```python
from build123d import *

# Parameters (mm, degrees)
EXTRUDE1_DEPTH     = 1.2
SKETCH3_R          = 6.35
EXTRUDE2_DEPTH     = 1.5
EXTRUDE3_DEPTH     = 0.75
SKETCH5_R          = 0.75
EXTRUDE4_DEPTH     = 0.3
SKETCH7_W          = 1.2
SKETCH7_H          = 1.2
SCALE1_SCALE       = 0.5
CUT_EXTRUDE1_DEPTH = 0.001


with BuildPart() as part:
    # Sketch1 → Revolve1 (revolve)
    with BuildSketch(Plane.XY):
        with BuildLine():
            Line((0, 0), (-6.25, 0))
            Line((-6.25, 0), (-6.25, 2.751471863))
            ThreePointArc((-6.25, 2.751471863), (-6.20432772, 2.981081922), (-6.074264069, 3.175735931))
            Line((-6.074264069, 3.175735931), (-5.674264069, 3.575735931))
            ThreePointArc((-5.674264069, 3.575735931), (-5.498528137, 4), (-5.674264069, 4.424264069))
            Line((-5.674264069, 4.424264069), (-6.074264069, 4.824264069))
            ThreePointArc((-6.074264069, 4.824264069), (-6.20432772, 5.018918078), (-6.25, 5.248528137))
            Line((-6.25, 5.248528137), (-6.25, 10.6))
            ThreePointArc((-6.25, 10.6), (-6.132842712, 10.882842712), (-5.85, 11))
            Line((-5.85, 11), (0, 11))
            Line((0, 11), (0, 0))
        make_face()
    revolve(axis=Axis((0, 11, 0), (0, -1, 0)))

    # Sketch2 → Extrude1 (add)
    with BuildSketch(Plane.XZ):
        with BuildLine():
            Line((-6.5, 5.5), (-5.5, 6.5))
            Line((-5.5, 6.5), (-1, 6.5))
            Line((-1, 6.5), (-1, 1.6))
            Line((-1, 1.6), (1, 1.6))
            Line((1, 1.6), (1, 6.5))
            Line((1, 6.5), (5.5, 6.5))
            Line((5.5, 6.5), (6.5, 5.5))
            Line((6.5, 5.5), (6.5, -5.5))
            ThreePointArc((6.5, -5.5), (6.207106781, -6.207106781), (5.5, -6.5))
            Line((5.5, -6.5), (1, -6.5))
            Line((1, -6.5), (1, -1.6))
            Line((1, -1.6), (-1, -1.6))
            Line((-1, -1.6), (-1, -6.5))
            Line((-1, -6.5), (-5.5, -6.5))
            ThreePointArc((-5.5, -6.5), (-6.207106781, -6.207106781), (-6.5, -5.5))
            Line((-6.5, -5.5), (-6.5, 5.5))
        make_face()
    extrude(amount=EXTRUDE1_DEPTH)

    # Sketch3 → Extrude2 (add)
    with BuildSketch(Plane(origin=(0, 0, 0), x_dir=(1, 0, 0), z_dir=(0, 1, 0))):
        with BuildLine():
            Line((5.5, -6.5), (-5.5, -6.5))
            Line((-5.5, -6.5), (-6.5, -5.5))
            Line((-6.5, -5.5), (-6.5, 5.5))
            ThreePointArc((-6.5, 5.5), (-6.207106781, 6.207106781), (-5.5, 6.5))
            Line((-5.5, 6.5), (5.5, 6.5))
            ThreePointArc((5.5, 6.5), (6.207106781, 6.207106781), (6.5, 5.5))
            Line((6.5, 5.5), (6.5, -5.5))
            Line((6.5, -5.5), (5.5, -6.5))
        make_face()
        Circle(SKETCH3_R, mode=Mode.SUBTRACT)
    extrude(amount=EXTRUDE2_DEPTH)

    # Sketch4 → Extrude3 (cut)
    with BuildSketch(Plane(origin=(0, 1.5, 0), x_dir=(1, 0, 0), z_dir=(0, 1, 0))):
        with BuildLine():
            Line((-6.5, 0), (-6.35, 0))
            ThreePointArc((-6.35, 0), (0, -6.35), (6.35, 0))
            Line((6.35, 0), (6.5, 0))
            Line((6.5, 0), (6.5, -5.5))
            Line((6.5, -5.5), (5.5, -6.5))
            Line((5.5, -6.5), (-5.5, -6.5))
            Line((-5.5, -6.5), (-6.5, -5.5))
            Line((-6.5, -5.5), (-6.5, 0))
        make_face()
    extrude(amount=-EXTRUDE3_DEPTH, mode=Mode.SUBTRACT)

    # Sketch5 → Extrude4 (add)
    with BuildSketch(Plane.XZ.offset(1.2)):
        with Locations((-4, 4)):
            Circle(SKETCH5_R)
        with Locations((4, 4)):
            Circle(SKETCH5_R)
        with Locations((-4, -4)):
            Circle(SKETCH5_R)
        with Locations((4, -4)):
            Circle(SKETCH5_R)
    extrude(amount=EXTRUDE4_DEPTH)

    # Sweep1: sweep along a path in Sketch6
    with BuildLine(Plane(origin=(0, 0, 0), x_dir=(0, 0, -1), z_dir=(1, 0, 0))) as sweep1_path:
        Line((2.7, 0), (2.7, -0.05))
        ThreePointArc((2.7, -0.05), (3.051471863, -0.898528137), (3.9, -1.25))
        Line((3.9, -1.25), (6.85, -1.25))
    # Sketch7 → Sweep1 (sweep)
    with BuildSketch(Plane.XZ):
        with Locations((0, -2.7)):
            Rectangle(SKETCH7_W, SKETCH7_H)
    sweep1 = sweep(path=sweep1_path.line)

    # Mirror1: Sweep1 across plane
    add(sweep1.mirror(Plane.XY))


with BuildPart() as part_1:
    # Scale1: scaled about (0, 4.617982794, -0.053235297)
    add(part.part.scale(SCALE1_SCALE).moved(Location((0, 2.308991397, -0.026617649))))

    # Sketch8 → Cut-Extrude1 (cut)
    with BuildSketch(Plane(origin=(0, 7.808991397, 0), x_dir=(1, 0, 0), z_dir=(0, 1, 0))):
        with BuildLine():
            Line((-2.568194891, -1.373382352), (2.568194891, -1.373382352))
            ThreePointArc((2.568194891, -1.373382352), (0, -2.898382352), (-2.568194891, -1.373382352))
        make_face()
    extrude(amount=-CUT_EXTRUDE1_DEPTH, mode=Mode.SUBTRACT)


solid = part_1.part
```
Verification items for the finished model (mm, model axes). A direction names the side the tool comes from. Round coordinates to 2 decimals unless told otherwise and drop trailing zeros. Write each loop counter-clockwise with the first axis right and the second up, starting at its lowest first coordinate (ties: lowest second). Pieces come first, ordered by that corner, then holes. Notation, with made-up numbers: (68.5, 12.25) -> (114.5, 12.25) arc R28 ccw to (114.5, 42.25) -> close; hole circle Ø10 at (80, 40). An arc over 180 degrees is marked (long way). Write each question's results on one line, items separated by ' | '. Start each with the question number.
1. Depth check by flat-ended pin: P1, Ø0.6, axis at x = 2, z = -2, coming from the -Y side; P2, Ø2, axis at x = 0.5, z = -1.5, coming from the -Y side. Enter the tip coordinate at first touch or a pass-through.
2. Material ranges on probe 1 along X at (y, z) = (5, 0); probe 2 along Y at (x, z) = (0.25, 2.5); probe 3 along Y at (x, z) = (2, -0.75), recorded low to high. Write a range as from..to.
3. Set-up check for faces 5 (the flat face through (0, 1.709, 0)), 6 (the flat face through (0.3, 1.7, -2.3)), 7 (the cylindrical face through (-2.887, 3.006, 1.17)), 8 (the flat face through (-0.3, 1.7, 2.2)): record each of +Z, -Z, +X, -X, +Y, -Y from which the full face is reachable in a straight line by a thin tool's end or side.
4. Cross-section at B-B (x = 0). Count the separate pieces of the cut face and the enclosed holes in it, then the cut area to 3 significant figures.
5. Cross-section at A-A (y = 2.5). Enter the section's corners in (x, z) (3 decimals), then the cut area to 3 significant figures.
6. Cross-section at C-C (y = 5.5). Enter the section's corners in (x, z) (3 decimals).
7. Draft check along X on faces 1 (the flat face through (3.25, 2, 0)), 2 (the flat face through (0, 2.309, 2)), 3 (the flat face through (-0.3, 1.7, -2.2)), 4 (the flat face through (1, 2, 3.223)). Enter one of: +X half, -X half, draft (parallel to the pull), parting line (faces both ways), or undercut.
Solutions:
1) P1: stops at y = 1.56 | P2: stops at y = 1.38
2) probe 1: x = -3.12..3.12 | probe 2: y = 1.38..1.98, 2.31..7.81 | probe 3: y = 1.71..7.81
3) face 5: -Y | face 6: -Z, -Y | face 7: +Y | face 8: +Z, -Y
4) separate pieces: 3 | enclosed holes: 0 | area: 37.9 mm2
5) outline: (-3.25, -2.777) arc R0.5 ccw to (-2.75, -3.277) -> (2.75, -3.277) arc R0.5 ccw to (3.25, -2.777) -> (3.25, 2.723) -> (2.75, 3.223) -> (-2.75, 3.223) -> (-3.25, 2.723) -> close; circle Ø6.25 at (0, -0.027); hole circle Ø6.35 at (0, -0.027) | area: 40.9 mm2
6) outline: circle Ø6.25 at (0, -0.027)
7) face 1: +X half | face 2: undercut | face 3: undercut | face 4: draft
